from build123d import *

# Parameters (mm, degrees)
SKETCH1_R           = 11.5
SKETCH1_R_2         = 1.6
BOSS_EXTRUDE1_DEPTH = 2
SKETCH2_R           = 4.5
SKETCH2_R_2         = 1.6
BOSS_EXTRUDE2_DEPTH = 2.5
SKETCH3_R           = 3
CUT_EXTRUDE1_DEPTH  = 3.6


with BuildPart() as part:
    # Sketch1 → Boss-Extrude1 (new body)
    with BuildSketch(Plane(origin=(0, 0, 0), x_dir=(1, 0, 0), z_dir=(0, 1, 0))):
        with Locations(Location((0, 0, 0), (0, 0, 270))):
            Circle(SKETCH1_R)
        with Locations(Location((-4.949747468, 4.949747468, 0), (0, 0, 270))):
            Circle(SKETCH1_R_2, mode=Mode.SUBTRACT)
        with Locations(Location((4.949747468, 4.949747468, 0), (0, 0, 270))):
            Circle(SKETCH1_R_2, mode=Mode.SUBTRACT)
        with Locations(Location((4.949747468, -4.949747468, 0), (0, 0, 270))):
            Circle(SKETCH1_R_2, mode=Mode.SUBTRACT)
        with Locations(Location((-4.949747468, -4.949747468, 0), (0, 0, 270))):
            Circle(SKETCH1_R_2, mode=Mode.SUBTRACT)
        with Locations(Location((0, 0, 0), (0, 0, 270))):
            Circle(SKETCH1_R_2, mode=Mode.SUBTRACT)
    extrude(amount=BOSS_EXTRUDE1_DEPTH)

    # Sketch2 → Boss-Extrude2 (add)
    with BuildSketch(Plane(origin=(0, 2, 0), x_dir=(1, 0, 0), z_dir=(0, 1, 0))):
        with Locations(Location((0, 0, 0), (0, 0, 270))):
            Circle(SKETCH2_R)
        with Locations(Location((0, 0, 0), (0, 0, 270))):
            Circle(SKETCH2_R_2, mode=Mode.SUBTRACT)
    extrude(amount=BOSS_EXTRUDE2_DEPTH)

    # Sketch3 → Cut-Extrude1 (cut)
    with BuildSketch(Plane(origin=(0, 4.5, 0), x_dir=(1, 0, 0), z_dir=(0, 1, 0))):
        with Locations(Location((0, 0, 0), (0, 0, 270))):
            Circle(SKETCH3_R)
    extrude(amount=-CUT_EXTRUDE1_DEPTH, mode=Mode.SUBTRACT)


solid = part.part
Source: CAD feature listing. Evaluate the final solid. Frame: model axes, mm. A direction names the side the tool comes from. Give positions to 0.01 mm unless a question says otherwise; leave off trailing zeros. Write each loop counter-clockwise with the first axis right and the second up, starting at its lowest first coordinate (ties: lowest second). Pieces come first, ordered by that corner, then holes. Notation, with made-up numbers: M 68,0.5 L 126,0.5 A21 ccw 126,16.5 Z; hole C -6,56 d10. An arc over 180 degrees is marked long. Return JSON: item names as keys, results as strings. Group by question number.
1) Pull-direction query (Z, two-part tool) for faces 3 (the face through (-1.3, 0.9, 1.3)), 4 (the face through (-3, 4.5, 1)), 5 (the face through (9.7, 0.99, 6.18)), 6 (the face through (0.9, 2.73, 2.86)); classes: pulls with the +Z half, pulls with the -Z half, needs draft (parallel to the pull), parting line crosses it, or undercut.
2) Cut plane C-C, the plane z = -4. Output: boundary loops of the cut face in (x, y), plus the area to 3 significant figures.
3) Cut plane D-D, the plane x = 5.25. Output: boundary loops of the cut face in (y, z), plus the area to 3 significant figures.
4) Pin query (flat end, axial travel): P1, Ø3, axis at x = -5, z = -5.5, coming from the +Y side; P2, Ø1.8, axis at x = 1, z = 1, coming from the +Y side; P3, Ø1.5, axis at y = 2.5, z = -7.5, coming from the -X side. Return the tip coordinate at first contact, or that it passes through.
5) Cut plane B-B, the plane z = 0. Output: boundary loops of the cut face in (x, y), plus the area to 3 significant figures.
6) Material intervals for line 1 along X through (y, z) = (3.4, 0); line 2 along X through (y, z) = (0.4, 0); line 3 along Z through (x, y) = (0.5, 3.8), sorted ascending. Write a range as [from, to].
7) Cut plane A-A, the plane x = 0. Output: boundary loops of the cut face in (y, z), plus the area to 3 significant figures.
8) Set-up query: faces 1 (the face through (-0.97, 0.44, -1.27)), 2 (the face through (1.352, 3.232, 4.292)). Return all of +Z, -Z, +X, -X, +Y, -Y with unobstructed straight access to the full face (end or side cutting, diameter ignored); none if empty.
Recorded:
{
 "1": {"face 3": "undercut", "face 4": "needs draft", "face 5": "parting line crosses it", "face 6": "undercut"},
 "2": {"outline": "M -10.78,0 L -6.24,0 L -6.24,2 L -10.78,2 Z; M -3.66,0 L 3.66,0 L 3.66,2 L 2.06,2 L 2.06,4.5 L -2.06,4.5 L -2.06,2 L -3.66,2 Z; M 6.24,0 L 10.78,0 L 10.78,2 L 6.24,2 Z", "area": "43.1 mm²"},
 "3": {"outline": "M 0,-10.23 L 2,-10.23 L 2,-6.52 L 0,-6.52 Z; M 0,-3.38 L 2,-3.38 L 2,3.38 L 0,3.38 Z; M 0,6.52 L 2,6.52 L 2,10.23 L 0,10.23 Z", "area": "28.4 mm²"},
 "4": {"P1": "stops at y = 2", "P2": "stops at y = 0.9", "P3": "stops at x = -9.17"},
 "5": {"outline": "M -11.5,0 L -1.6,0 L -1.6,0.9 L -3,0.9 L -3,4.5 L -4.5,4.5 L -4.5,2 L -11.5,2 Z; M 1.6,0 L 11.5,0 L 11.5,2 L 4.5,2 L 4.5,4.5 L 3,4.5 L 3,0.9 L 1.6,0.9 Z", "area": "44.0 mm²"},
 "6": {"line 1": "x = [-4.5, -3], [3, 4.5]", "line 2": "x = [-11.5, -1.6], [1.6, 11.5]", "line 3": "z = [-4.47, -2.96], [2.96, 4.47]"},
 "7": {"outline": "M 0,-11.5 L 2,-11.5 L 2,-4.5 L 4.5,-4.5 L 4.5,-3 L 0.9,-3 L 0.9,-1.6 L 0,-1.6 Z; M 0,1.6 L 0.9,1.6 L 0.9,3 L 4.5,3 L 4.5,4.5 L 2,4.5 L 2,11.5 L 0,11.5 Z", "area": "44.0 mm²"},
 "8": {"face 1": "+Y, -Y", "face 2": "+Y"}
}
